Study the drawing (mm; zero at the part's minimum x, y, z) and answer. Coordinates: 2 decimals unless noted, no trailing zeros. Write each loop counter-clockwise with the first axis right and the second up, starting at its lowest first coordinate (ties: lowest second). Pieces come first, ordered by that corner, then holes. Notation, with made-up numbers: M -33.5,7.5 L -2.5,7.5 A27 cw -2.5,36.5 Z; hole C -28,48.25 d10. An arc over 180 degrees is marked long. Answer as CSV lines item,"result". Start each with the question number.
(1) A cutting plane is placed at B-B on z = 13.25. Give the vertices of the cut face in (x, y), then the cut area to 3 significant figures.
(2) A cutting plane is placed at A-A on x = 180. Give the vertices of the cut face in (y, z).
(3) A cutting plane is placed at D-D on y = 20. Give the vertices of the cut face in (x, z).
(4) Flat-ended cylindrical pins translate along their axes: P1, Ø5, axis at x = 227.5, y = 28.5, coming from the -Z side; P2, Ø9, axis at x = 189.5, y = 12, coming from the +Z side; P3, Ø6, axis at x = 225, z = 18, coming from the -Y side. Find the tip coordinate at first contact, or state that the pin passes through.
(5) A cutting plane is placed at C-C on y = 75. Give the vertices of the cut face in (x, z).
(6) Find the intervals of material crossed by L1, parallel to Y at x = 120, z = 16.25; L2, parallel to Y at x = 120, z = 9.5; L3, parallel to Z at x = 281, y = 64, in increasing order. Write a range as [from, to].
(7) The mould has two halves that part along X. Classify the marked faces 1 and 2: released by +X, released by -X, zero draft, split by the parting line, or undercut.
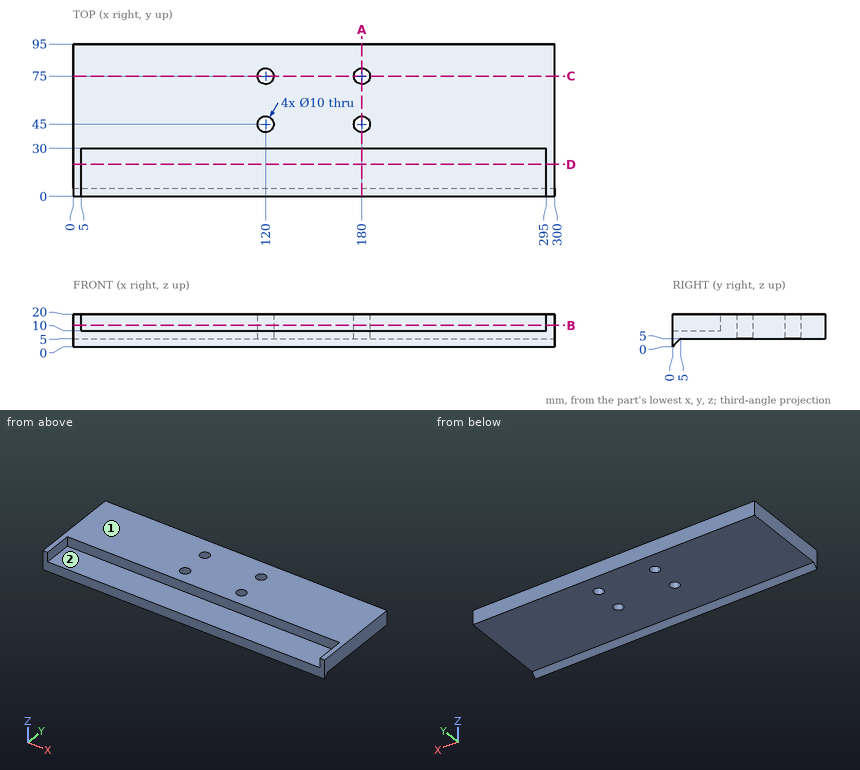
Here are the results:
1,outline,"M 0,0 L 5,0 L 5,30 L 295,30 L 295,0 L 300,0 L 300,95 L 0,95 Z; hole C 120,45 d10; hole C 120,75 d10; hole C 180,45 d10; hole C 180,75 d10"
1,area,"19,500 mm^2"
2,outline,"M 0,0 L 5,5 L 40,5 L 40,20 L 30,20 L 30,10 L 0,10 Z; M 50,5 L 70,5 L 70,20 L 50,20 Z; M 80,5 L 95,5 L 95,20 L 80,20 Z"
3,outline,"M 0,5 L 300,5 L 300,20 L 295,20 L 295,10 L 5,10 L 5,20 L 0,20 Z"
4,P1,"stops at z = 5"
4,P2,"stops at z = 10"
4,P3,"stops at y = 30"
5,outline,"M 0,5 L 115,5 L 115,20 L 0,20 Z; M 125,5 L 175,5 L 175,20 L 125,20 Z; M 185,5 L 300,5 L 300,20 L 185,20 Z"
6,L1,"y = [30, 40], [50, 70], [80, 95]"
6,L2,"y = [0, 40], [50, 70], [80, 95]"
6,L3,"z = [5, 20]"
7,face 1,"zero draft"
7,face 2,"undercut"
